Autodesk Inventor part; units mm, degrees
ref_plane "YZ Plane" through (0, 0, 0) normal (1, 0, 0) x (0, 1, 0)
ref_plane "XZ Plane" through (0, 0, 0) normal (0, 1, 0) x (-1, 0, 0)
ref_plane "XY Plane" through (0, 0, 0) normal (0, 0, 1) x (1, 0, 0)
sketch "Sketch1" plane through (0, 0, 0) normal (0, 0, 1) x (1, 0, 0)
  line L0 (-12.5, -70) -> (12.5, -70)
  line L1 (12.5, -70) -> (12.5, 70)
  line L2 (12.5, 70) -> (-12.5, 70)
  line L3 (-12.5, 70) -> (-12.5, -70)
  line L4 (-12.5, -70) -> (12.5, 70) construction
  line L5 (12.5, -70) -> (-12.5, 70) construction
  line L6 (0, 70) -> (0, -70)
  line L7 (12.5, 29.75) -> (15.6, 29.75)
  line L8 (15.6, 29.75) -> (15.6, -29.75)
  line L9 (15.6, -29.75) -> (12.5, -29.75)
  line L10 (12.5, -29.75) -> (12.5, 29.75)
  line L11 (-12.5, 29.75) -> (-15.6, 29.75)
  line L12 (-15.6, 29.75) -> (-15.6, -29.75)
  line L13 (-15.6, -29.75) -> (-12.5, -29.75)
  line L14 (-12.5, -29.75) -> (-12.5, 29.75)
  line L15 (-12.5, 70) -> (12.5, 70)
  line L16 (12.5, 70) -> (12.5, 90)
  line L17 (12.5, 90) -> (-12.5, 90)
  line L18 (-12.5, 90) -> (-12.5, 70)
  point P0 (0, 0)
  point P1 (15.6, 0)
  point P2 (0, 0)
  point P3 (-15.6, 0)
  point P4 (-12.5, 29.75)
  point P5 (-12.5, -29.75)
  point P6 (12.5, -29.75)
  dimension "d0" = 140
  dimension "d1" = 59.5
  dimension "d2" = 3.1
  dimension "d3" = 25
  dimension "d5" = 20
extrude "Plate1" add sketch "Sketch1" along normal mid plane 3
equation "\"d4\" = Thickness"
equation "\"BendRadius\" = Thickness"
equation "\"BendReliefWidth\" = Thickness"
equation "\"BendReliefDepth\" = 0.5 * Thickness"
equation "\"CornerReliefSize\" = 4 * Thickness"
equation "\"MinimumRemnant\" = 2 * Thickness"
equation "\"TransitionRadius\" = BendRadius"
equation "\"JacobiRadiusSize\" = BendRadius"
equation "\"GapSize\" = Thickness"
properties part number "Motor Fixation .2"
Verification items for the finished model (mm, model axes). A direction names the side the tool comes from. Give positions to 0.01 mm unless a question says otherwise; leave off trailing zeros. Order: outer loops, then holes, each group sorted by start corner. A loop starts at its lowest first (then second) coordinate and runs counter-clockwise, first axis right, second up. Notation, with made-up numbers: (-39.75, 27.5) -> (15.25, 27.5) arc R24 cw to (15.25, 56.5) -> close; hole circle Ø7 at (89, 62). An arc over 180 degrees is marked (long way). Answer as CSV lines item,"result".
Q1. Sectioned sample at A-A on z = -0.2. Record the cut outline in (x, y), plus the area to 3 significant figures.
Solutions:
outline,"(-15.6, -29.75) -> (-12.5, -29.75) -> (-12.5, -70) -> (12.5, -70) -> (12.5, -29.75) -> (15.6, -29.75) -> (15.6, 29.75) -> (12.5, 29.75) -> (12.5, 90) -> (-12.5, 90) -> (-12.5, 29.75) -> (-15.6, 29.75) -> close"
area,"4,370 mm²"
Q2. Scan lines: probe 1 along X at (y, z) = (33, -0.2); probe 2 along Y at (x, z) = (14, 0.65). Record each from-to range of solid material in increasing order.
Solutions:
probe 1,"x = -12.5 to 12.5"
probe 2,"y = -29.75 to 29.75"
Q3. Access from +Z, -Z, +X, -X, +Y, -Y to the whole of each face (thin tool, end or side, straight path). Record for faces 1 (the flat face through (0, 90, 0)), 2 (the flat face through (12.5, -50, 0)), 3 (the flat face through (-12.5, 60, 0)), 4 (the flat face through (-12.5, -50, 0)), 5 (the flat face through (12.5, 59, 0)).
Solutions:
face 1,"+Z, -Z, +X, -X, +Y"
face 2,"+Z, -Z, +X, -Y"
face 3,"+Z, -Z, -X, +Y"
face 4,"+Z, -Z, -X, -Y"
face 5,"+Z, -Z, +X, +Y"
Q4. Depth check by flat-ended pin: pin 1 (1.5 mm diameter, centred on y = -51.5, z = 0, fed in from +X); pin 2 (0.9 mm diameter, centred on x = 15, z = 0, fed in from +Y); pin 3 (0.9 mm diameter, centred on x = -14.5, z = -0.5, fed in from -Y). Enter the tip coordinate at first touch or a pass-through.
Solutions:
pin 1,"stops at x = 12.5"
pin 2,"stops at y = 29.75"
pin 3,"stops at y = -29.75"
Q5. Sectioned sample at C-C on x = -14. Record the cut outline in (y, z), plus the area to 4 significant figures.
Solutions:
outline,"(-29.75, -1.5) -> (29.75, -1.5) -> (29.75, 1.5) -> (-29.75, 1.5) -> close"
area,"178.5 mm²"
Q6. Sectioned sample at B-B on y = 38. Record the cut outline in (x, z).
Solutions:
outline,"(-12.5, -1.5) -> (12.5, -1.5) -> (12.5, 1.5) -> (-12.5, 1.5) -> close"
